Here's how the part is built. I have some questions about the finished solid (model axes, mm). Face numbers are marked on the shaded views. A direction names the side the tool comes from. Give positions to 0.01 mm unless a question says otherwise; leave off trailing zeros. Loops run counter-clockwise (first coordinate to the right, second up) from the corner with the lowest first, then second, coordinate; pieces in that order, holes last.
Q1. I'm going to push flat-ended pins straight in: P1, Ø1, axis at y = 1.5, z = 9.5, coming from the -X side; P2, Ø2.5, axis at x = -1.5, y = -2, coming from the +Z side; P3, Ø3, axis at x = 0, z = 7, coming from the +Y side. Where does each tip first touch, or does it pass through?
Q2. For the marked faces 4 and 5, which set-ups out of +Z, -Z, +X, -X, +Y, -Y let a thin tool reach every point of the face, with its end or its side?
Q3. Thinking about a two-plate mould opening in Y: for the marked faces 1, 2 and 3, which applies, pulls with the +Y half, pulls with the -Y half, needs draft (parallel to the pull), parting line crosses it, or undercut?
Q4. Suppose I cut it at B-B (x = 0). List the corners of the cut face in (y, z) for me, and give its area (3 significant figures).
Q5. Suppose I cut it at C-C (y = -0.5). List the corners of the cut face in (x, z) for me.
Q6. I need wall thicknesses on probe 1 along X at (y, z) = (-2.25, 8.25); probe 2 along X at (y, z) = (0, 0.5); probe 3 along Y at (x, z) = (-3.5, 11). Which ranges of each line are inside material? Lowest first, please.
Q7. Suppose I cut it at A-A (z = 8). List the corners of the cut face in (x, y) for me (3 decimals), and give its area (3 significant figures).
```python
from build123d import *

# Parameters (mm, degrees)
F0_R     = 1.6
F1_DEPTH = 12
F5_DEPTH = 4
F6_R     = 4
F7_DEPTH = 25


with BuildPart() as f1:
    # F0 (on Top) → F1 (new body)
    with BuildSketch(Plane.XY):
        with BuildLine():
            ThreePointArc((6.5812443787, -3.5968350571), (5.3517467882, -1.2683872891), (7.4954714157, 0.260592127))
            ThreePointArc((7.4954714157, 0.260592127), (7.4827308748, 0.5086635974), (7.4617823733, 0.7561771044))
            ThreePointArc((7.4617823733, 0.7561771044), (5.130860376, 1.9809774864), (6.0339352218, 4.4543939811))
            ThreePointArc((6.0339352218, 4.4543939811), (5.8831174869, 4.6517661845), (5.7258464401, 4.8440357704))
            ThreePointArc((5.7258464401, 4.8440357704), (3.1108378152, 4.5357125226), (2.456599692, 7.0862626224))
            ThreePointArc((2.456599692, 7.0862626224), (2.2205890006, 7.1637269972), (1.9821424996, 7.2333333333))
            ThreePointArc((1.9821424996, 7.2333333333), (0, 5.5), (-1.9821424996, 7.2333333333))
            ThreePointArc((-1.9821424996, 7.2333333333), (-2.490988884, 7.0742472659), (-2.9872482232, 6.8794148045))
            Line((-2.9872482232, 6.8794148045), (-2.7759390923, 6.426260911))
            Line((-2.7759390923, 6.426260911), (-3.1384622071, 6.2572136063))
            Line((-3.1384622071, 6.2572136063), (-3.349771338, 6.7103674999))
            ThreePointArc((-3.349771338, 6.7103674999), (-3.8180110168, 6.4554466829), (-4.2669581658, 6.1679062907))
            ThreePointArc((-4.2669581658, 6.1679062907), (-4.2132444372, 3.5353318533), (-6.8151514446, 3.1310877961))
            ThreePointArc((-6.8151514446, 3.1310877961), (-6.915100354, 2.9036850887), (-7.0074639483, 2.6730972696))
            ThreePointArc((-7.0074639483, 2.6730972696), (-5.4741653769, 0.5324597889), (-7.3912498308, -1.2725666735))
            ThreePointArc((-7.3912498308, -1.2725666735), (-7.3450546632, -1.5166317925), (-7.2908025549, -1.7590332871))
            ThreePointArc((-7.2908025549, -1.7590332871), (-4.8155702722, -2.6571192961), (-5.3756065246, -5.2299956494))
            ThreePointArc((-5.3756065246, -5.2299956494), (-5.1994656152, -5.4051417481), (-5.0176213056, -5.5743588361))
            ThreePointArc((-5.0176213056, -5.5743588361), (-2.4683954911, -4.9149795218), (-1.4750068347, -7.3535266939))
            ThreePointArc((-1.4750068347, -7.3535266939), (-1.2306839919, -7.3983387941), (-0.9850111866, -7.4350355051))
            ThreePointArc((-0.9850111866, -7.4350355051), (0.7443221486, -5.4494022185), (2.9428039897, -6.8985436636))
            ThreePointArc((2.9428039897, -6.8985436636), (3.1696369631, -6.7973084028), (3.3929930968, -6.6886170353))
            ThreePointArc((3.3929930968, -6.6886170353), (3.6960432331, -4.0729920721), (6.3287206193, -4.0245863543))
            ThreePointArc((6.3287206193, -4.0245863543), (6.4585247429, -3.8128018759), (6.5812443787, -3.5968350571))
        make_face()
        Circle(F0_R, mode=Mode.SUBTRACT)
    extrude(amount=F1_DEPTH)

    # F4 (on offset) → F5 (cut)
    with BuildSketch(Plane(origin=(0, 0, 1.5), x_dir=(1, 0, 0), z_dir=(0, 0, -1))):
        Polygon((3.4640966662, -0.0058555579), (1.737119395, 2.9970679351), (-1.7269772711, 3.002923493), (-3.4640966662, 0.0058555579), (-1.737119395, -2.9970679351), (1.7269772711, -3.002923493), align=None)
    extrude(amount=-F5_DEPTH, mode=Mode.SUBTRACT)

    # F6 (on offset) → F7 (cut)
    with BuildSketch(Plane(origin=(0, 0, 5.5), x_dir=(1, 0, 0), z_dir=(0, 0, -1))):
        Circle(F6_R)
    extrude(amount=-F7_DEPTH, mode=Mode.SUBTRACT)


solid = f1.part
```
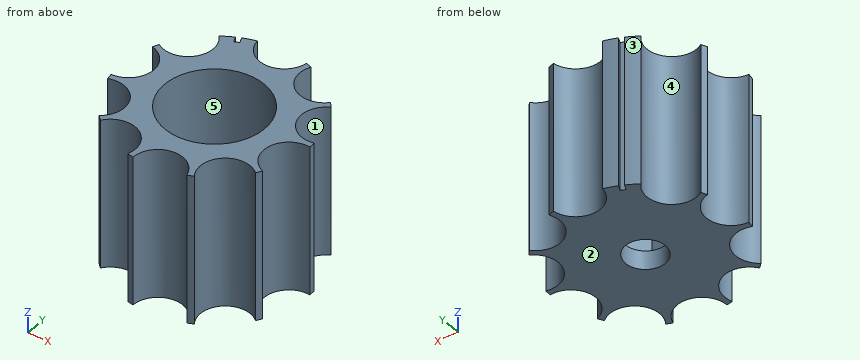
Solutions:
1. P1: stops at x = -5.92
1. P2: stops at z = 5.5
1. P3: stops at y = 6.18
2. face 4: +Z, -Z
2. face 5: +Z
3. face 1: undercut
3. face 2: needs draft
3. face 3: pulls with the +Y half
4. outline: (-5.71, 0) - (-1.6, 0) - (-1.6, 1.5) - (-3, 1.5) - (-3, 5.5) - (-4, 5.5) - (-4, 12) - (-5.71, 12) - close; (1.6, 0) - (5.5, 0) - (5.5, 12) - (4, 12) - (4, 5.5) - (3, 5.5) - (3, 1.5) - (1.6, 1.5) - close
4. area: 53.7 mm2
5. outline: (-5.88, 0) - (-1.52, 0) - (-1.52, 1.5) - (-3.18, 1.5) - (-3.18, 5.5) - (-3.97, 5.5) - (-3.97, 12) - (-5.88, 12) - close; (1.52, 0) - (5.72, 0) - (5.72, 12) - (3.97, 12) - (3.97, 5.5) - (3.17, 5.5) - (3.17, 1.5) - (1.52, 1.5) - close
6. probe 1: x = -5.11 to -3.31, 3.31 to 5.37
6. probe 2: x = -5.6 to -1.6, 1.6 to 6.29
6. probe 3: y = -4.71 to -1.94, 1.94 to 6.63
7. outline: (-7.391, -1.273) arc R7.5 ccw to (-7.291, -1.759) arc R2 cw to (-5.376, -5.23) arc R7.5 ccw to (-5.018, -5.574) arc R2 cw to (-1.475, -7.354) arc R7.5 ccw to (-0.985, -7.435) arc R2 cw to (2.943, -6.899) arc R7.5 ccw to (3.393, -6.689) arc R2 cw to (6.329, -4.025) arc R7.5 ccw to (6.581, -3.597) arc R2 cw to (7.495, 0.261) arc R7.5 ccw to (7.462, 0.756) arc R2 cw to (6.034, 4.454) arc R7.5 ccw to (5.726, 4.844) arc R2 cw to (2.457, 7.086) arc R7.5 ccw to (1.982, 7.233) arc R2 cw to (-1.982, 7.233) arc R7.5 ccw to (-2.987, 6.879) - (-2.776, 6.426) - (-3.138, 6.257) - (-3.35, 6.71) arc R7.5 ccw to (-4.267, 6.168) arc R2 cw to (-6.815, 3.131) arc R7.5 ccw to (-7.007, 2.673) arc R2 cw to start; hole circle Ø8 at (0, 0)
7. area: 67.0 mm2
